from build123d import *

# Parameters (mm, degrees)
SKETCH1_R           = 18
BOSS_EXTRUDE1_DEPTH = 35
SKETCH2_R           = 10
BOSS_EXTRUDE2_DEPTH = 3
SKETCH3_R           = 3
BOSS_EXTRUDE3_DEPTH = 15
SKETCH4_R           = 1.5
CUT_EXTRUDE1_DEPTH  = 15


with BuildPart() as part:
    # Sketch1 → Boss-Extrude1 (new body)
    with BuildSketch(Plane.XY):
        Circle(SKETCH1_R)
    extrude(amount=BOSS_EXTRUDE1_DEPTH)

    # Sketch2 → Boss-Extrude2 (add)
    with BuildSketch(Plane.XY.offset(35)):
        Circle(SKETCH2_R)
    extrude(amount=BOSS_EXTRUDE2_DEPTH)

    # Sketch3 → Boss-Extrude3 (add)
    with BuildSketch(Plane.XY.offset(38)):
        Circle(SKETCH3_R)
    extrude(amount=BOSS_EXTRUDE3_DEPTH)

    # Sketch4 → Cut-Extrude1 (cut)
    with BuildSketch(Plane.XY.offset(35)):
        with Locations((0, 15)):
            Circle(SKETCH4_R)
        with Locations((12.990381057, -7.5)):
            Circle(SKETCH4_R)
        with Locations((-12.990381057, -7.5)):
            Circle(SKETCH4_R)
    extrude(amount=-CUT_EXTRUDE1_DEPTH, mode=Mode.SUBTRACT)


solid = part.part
Geometry: final body of the model. Coordinates: model frame, mm. A direction names the side the tool comes from. Round coordinates to 2 decimals unless told otherwise and drop trailing zeros. Order: outer loops, then holes, each group sorted by start corner. A loop starts at its lowest first (then second) coordinate and runs counter-clockwise, first axis right, second up.
Q1. Access query for faces 1 (the face through (0, 0, 53)), 2 (the face through (-3, 0, 45)). Directions: +Z, -Z, +X, -X, +Y, -Y. A direction counts if a zero-diameter tool reaches every point of the face in a straight line with its end or side. Return the directions, or none.
Result sheet:
face 1: +Z, +X, -X, +Y, -Y
face 2: +Z
Q2. Section A-A, the plane y = 0. Output: boundary loops of the cut face in (x, z).
Result sheet:
outline: (-18, 0) - (18, 0) - (18, 35) - (10, 35) - (10, 38) - (3, 38) - (3, 53) - (-3, 53) - (-3, 38) - (-10, 38) - (-10, 35) - (-18, 35) - close
Q3. Mould query, pull axis X, two halves, no side actions, for faces 3 (the face through (2.1, 2.4, 38)), 4 (the face through (-2.343, 17.847, 17.255)), 5 (the face through (-1.11, 16.01, 27.6)). Classes: released by +X, released by -X, zero draft, split by the parting line, or undercut.
Result sheet:
face 3: zero draft
face 4: split by the parting line
face 5: undercut
Q4. Pin query (flat end, axial travel): pin 1 (3.5 mm diameter, centred on x = -13, y = -7.5, fed in from +Z); pin 2 (6 mm diameter, centred on x = -10.5, z = 32.5, fed in from -Y); pin 3 (10 mm diameter, centred on x = -8, z = 29.5, fed in from +Y). Return the tip coordinate at first contact, or that it passes through.
Result sheet:
pin 1: stops at z = 35
pin 2: stops at y = -16.36
pin 3: stops at y = 17.75
Q5. Section D-D, the plane y = 8. Output: boundary loops of the cut face in (x, z), and give its area (3 significant figures).
Result sheet:
outline: (-16.12, 0) - (16.12, 0) - (16.12, 35) - (6, 35) - (6, 38) - (-6, 38) - (-6, 35) - (-16.12, 35) - close
area: 1,160 mm2
Q6. Section C-C, the plane z = 10.5. Output: boundary loops of the cut face in (x, y).
Result sheet:
outline: circle Ø36 at (0, 0)
Q7. Material intervals for probe 1 along X at (y, z) = (-7, 31); probe 2 along Y at (x, z) = (0, 24.5); probe 3 along Z at (x, y) = (4, 9.5), sorted ascending.
Result sheet:
probe 1: x = -16.58 to -14.4, -11.58 to 11.58, 14.4 to 16.58
probe 2: y = -18 to 13.5, 16.5 to 18
probe 3: z = 0 to 35
Q8. Section B-B, the plane x = 0. Output: boundary loops of the cut face in (y, z).
Result sheet:
outline: (-18, 0) - (18, 0) - (18, 35) - (16.5, 35) - (16.5, 20) - (13.5, 20) - (13.5, 35) - (10, 35) - (10, 38) - (3, 38) - (3, 53) - (-3, 53) - (-3, 38) - (-10, 38) - (-10, 35) - (-18, 35) - close
